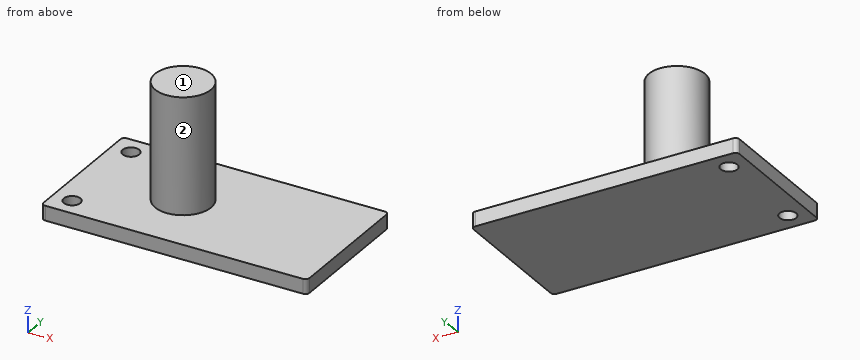
from build123d import *

# Parameters (mm, degrees)
MEASURED_ENCODER_PCB_DEPTH         = 1.78
SKETCH_2_R                         = 1.015
MEASURED_ENCODER_MOUNT_HOLES_DEPTH = 2
SHAFT_CLEARANCE_REFERENCE_START    = 1.78
SKETCH_3_R                         = 3.405
SHAFT_CLEARANCE_REFERENCE_DEPTH    = 14.12


with BuildPart() as part:
    # 草图1 → Measured_encoder_PCB (new body)
    with BuildSketch(Plane.XY):
        with BuildLine():
            Line((0.5, 0), (31.8, 0))
            ThreePointArc((31.8, 0), (32.153553391, 0.146446609), (32.3, 0.5))
            Line((32.3, 0.5), (32.3, 16.42))
            ThreePointArc((32.3, 16.42), (32.153553391, 16.773553391), (31.8, 16.92))
            Line((31.8, 16.92), (0.5, 16.92))
            ThreePointArc((0.5, 16.92), (0.146446609, 16.773553391), (0, 16.42))
            Line((0, 16.42), (0, 0.5))
            ThreePointArc((0, 0.5), (0.146446609, 0.146446609), (0.5, 0))
        make_face()
    extrude(amount=MEASURED_ENCODER_PCB_DEPTH)

    # 草图2 → Measured_encoder_mount_holes (cut)
    with BuildSketch(Plane.XY):
        with Locations((2.365, 2.365)):
            Circle(SKETCH_2_R)
        with Locations((2.365, 14.555)):
            Circle(SKETCH_2_R)
    extrude(amount=MEASURED_ENCODER_MOUNT_HOLES_DEPTH, mode=Mode.SUBTRACT)

    # 草图3 → Shaft_clearance_reference (add)
    with BuildSketch(Plane.XY.offset(SHAFT_CLEARANCE_REFERENCE_START)):
        with Locations((12.275, 8.46)):
            Circle(SKETCH_3_R)
    extrude(amount=SHAFT_CLEARANCE_REFERENCE_DEPTH)


solid = part.part
The listing builds one solid part. Answer for the finished solid, in the listing's coordinates (mm). Face numbers are marked on the shaded views. A direction names the side the tool comes from. Round coordinates to 2 decimals unless told otherwise and drop trailing zeros. Loops run counter-clockwise (first coordinate to the right, second up) from the corner with the lowest first, then second, coordinate; pieces in that order, holes last. Notation, with made-up numbers: M -2,-28 L 5,-28 A31 cw 5,8 Z; hole C 44.5,-31.75 d5. An arc over 180 degrees is marked long. Write each question's results on one line, items separated by ' | '. Start each with the question number.
1) Find section C-C on z = 8.75. Write down the section's boundary in (x, y) (3 decimals).
2) Find section B-B on y = 8.46. Write down the section's boundary in (x, z).
3) Which of the six approach directions +Z, -Z, +X, -X, +Y, -Y give full straight-line access (tool end or side, diameter ignored) to the marked faces 1 and 2?
4) Straight lines are drawn through the part: probe 1 along Z at (x, y) = (21.5, 3.75); probe 2 along X at (y, z) = (5.75, 4.75); probe 3 along X at (y, z) = (6.25, 14.5). For each, find the intervals that lie inside material, in ascending order.
5) Find section D-D on x = 10. Write down the section's boundary in (y, z), plus the area to 3 significant figures.
6) Find section A-A on x = 2. Write down the section's boundary in (y, z).
7) Each of these flat-tipped pins is pushed along its axis until it touches: pin 1 (2.5 mm diameter, centred on x = 2.365, y = 2.365, fed in from +Z); pin 2 (8 mm diameter, centred on x = 20, z = 6.5, fed in from -Y). Where does it stop, or does it pass through?
Final values:
1) outline: C 12.275,8.46 d6.81
2) outline: M 0,0 L 32.3,0 L 32.3,1.78 L 15.68,1.78 L 15.68,15.9 L 8.87,15.9 L 8.87,1.78 L 0,1.78 Z
3) face 1: +Z, +X, -X, +Y, -Y | face 2: +Z
4) probe 1: 0 to 1.78 | probe 2: 10.21 to 14.34 | probe 3: 9.68 to 14.87
5) outline: M 0,0 L 16.92,0 L 16.92,1.78 L 10.99,1.78 L 10.99,15.9 L 5.93,15.9 L 5.93,1.78 L 0,1.78 Z | area: 102 mm²
6) outline: M 0,0 L 1.42,0 L 1.42,1.78 L 0,1.78 Z; M 3.31,0 L 13.61,0 L 13.61,1.78 L 3.31,1.78 Z; M 15.5,0 L 16.92,0 L 16.92,1.78 L 15.5,1.78 Z
7) pin 1: z = 1.78 | pin 2: through
